Here's how the part is built. I have some questions about the finished solid (model axes, mm). A direction names the side the tool comes from. Coordinates: 2 decimals unless noted, no trailing zeros. Write each loop counter-clockwise with the first axis right and the second up, starting at its lowest first coordinate (ties: lowest second). Pieces come first, ordered by that corner, then holes. Notation, with made-up numbers: M 39.5,-23 L 57.5,-23 A18 cw 57.5,5 Z; hole C -17,88 d10. An arc over 180 degrees is marked long. Use a Markdown table: item, result.
```python
from build123d import *

# Parameters (mm, degrees)
F0_R     = 25
F0_R_2   = 5
F0_R_3   = 2.5
F0_R_4   = 3.5
F1_DEPTH = 19
F2_T     = -4
F3_DEPTH = 25
F4_R     = 25
F5_DEPTH = 2


# Not quite as in the source:
# - a feature names something its author has since deleted; it is built from what else it names


with BuildPart() as f1:
    # F0 (on Top) → F1 (new body)
    with BuildSketch(Plane.XY):
        Circle(F0_R)
        with Locations((-12.990381, -7.5)):
            Circle(F0_R_2, mode=Mode.SUBTRACT)
        with Locations((0, -15)):
            Circle(F0_R_3, mode=Mode.SUBTRACT)
        with Locations((12.990381, -7.5)):
            Circle(F0_R_2, mode=Mode.SUBTRACT)
        with Locations((-12.990381, 7.5)):
            Circle(F0_R_3, mode=Mode.SUBTRACT)
        Circle(F0_R_4, mode=Mode.SUBTRACT)
        with Locations((12.990381, 7.5)):
            Circle(F0_R_3, mode=Mode.SUBTRACT)
        with Locations((0, 15)):
            Circle(F0_R_2, mode=Mode.SUBTRACT)
        Circle(F0_R_4)
        with Locations((-12.990381, 7.5)):
            Circle(F0_R_3)
        with Locations((12.990381, 7.5)):
            Circle(F0_R_3)
        with Locations((0, -15)):
            Circle(F0_R_3)
    extrude(amount=F1_DEPTH)

    # F2
    f2_openings = [f1.faces().sort_by_distance(p)[0] for p in [
        (0, 0, 19),
    ]]
    offset(amount=F2_T, openings=f2_openings)

    # F0 (on Top) → F3 (cut)
    with BuildSketch(Plane.XY):
        with Locations((-12.990381, 7.5)):
            Circle(F0_R_3)
        Circle(F0_R_4)
        with Locations((12.990381, 7.5)):
            Circle(F0_R_3)
        with Locations((0, -15)):
            Circle(F0_R_3)
    extrude(amount=F3_DEPTH, mode=Mode.SUBTRACT)

    # F4 (on face) → F5 (join)
    with BuildSketch(Plane.XY.offset(19)):
        Circle(F4_R)
        with BuildLine():
            ThreePointArc((-20.78461, -3), (-18.186533, 10.5), (-7.794229, 19.5))
            ThreePointArc((-7.794229, 19.5), (0, 6), (7.794229, 19.5))
            ThreePointArc((7.794229, 19.5), (18.186533, 10.5), (20.78461, -3))
            ThreePointArc((20.78461, -3), (5.196152, -3), (12.990381, -16.5))
            ThreePointArc((12.990381, -16.5), (0, -21), (-12.990381, -16.5))
            ThreePointArc((-12.990381, -16.5), (-5.196152, -3), (-20.78461, -3))
        make_face(mode=Mode.SUBTRACT)
    extrude(amount=F5_DEPTH)


solid = f1.part
```
1. I need wall thicknesses on probe 1 along Y at (x, z) = (0, 1); probe 2 along Y at (x, z) = (14.5, 12.5); probe 3 along Y at (x, z) = (14, 1.5). Which ranges of each line are inside material? Lowest first, please.
Answers follow:
| item | result |
|---|---|
| probe 1 | y = -25 to -17.5, -12.5 to -3.5, 3.5 to 10, 20 to 25 |
| probe 2 | y = -20.37 to -12.27, -2.73 to 1.37, 15.19 to 20.37 |
| probe 3 | y = -20.71 to -12.4, -2.6 to 5.21, 9.79 to 20.71 |
2. Suppose I cut it at D-D on y = 7.5. Write out the boundary of the cut face in (x, z), and give its area (3 significant figures).
Answers follow:
| item | result |
|---|---|
| outline | M -23.85,0 L -15.49,0 L -15.49,4 L -19.62,4 L -19.62,21 L -23.85,21 Z; M -10.49,0 L 10.49,0 L 10.49,4 L 4.97,4 L 4.97,21 L -4.97,21 L -4.97,4 L -10.49,4 Z; M 15.49,0 L 23.85,0 L 23.85,21 L 19.62,21 L 19.62,4 L 15.49,4 Z |
| area | 464 mm2 |
3. We'd pull the mould along X, two halves only. Please class faces 1 (the face through (12.45, 5.06, 1.97)), 2 (the face through (12.339, -2.543, 9.367)), 3 (the face through (5, 0, 0)), 4 (the face through (23.846, 7.509, 10.353)): +X half, -X half, draft (parallel to the pull), parting line (faces both ways), or undercut.
Answers follow:
| item | result |
|---|---|
| face 1 | undercut |
| face 2 | undercut |
| face 3 | draft |
| face 4 | parting line |
4. Suppose I cut it at C-C on y = -15. Write out the boundary of the cut face in (x, z), and give its area (3 significant figures).
Answers follow:
| item | result |
|---|---|
| outline | M -20,0 L -2.5,0 L -2.5,4 L -8.02,4 L -8.02,21 L -20,21 Z; M 2.5,0 L 20,0 L 20,21 L 8.02,21 L 8.02,4 L 2.5,4 Z |
| area | 547 mm2 |
5. Suppose I cut it at A-A on z = 8.5. Write out the boundary of the cut face in (x, y), and give its area (3 significant figures).
Answers follow:
| item | result |
|---|---|
| outline | C 0,0 d50; hole M -20.78,-3 A9 cw long -12.99,-16.5 A21 ccw 12.99,-16.5 A9 cw long 20.78,-3 A21 ccw 7.79,19.5 A9 cw long -7.79,19.5 A21 ccw Z; hole C -12.99,-7.5 d10; hole C 0,15 d10; hole C 12.99,-7.5 d10 |
| area | 1,000 mm2 |
6. Which directions (+Z, -Z, +X, -X, +Y, -Y) give clear straight access to the entire face, cutting with the end or side of a thin tool? Please do faces 5 (the face through (3.233, -1.341, 1.972)), 6 (the face through (0, 4, 4)), 7 (the face through (-13, -7, 19)).
Answers follow:
| item | result |
|---|---|
| face 5 | +Z, -Z |
| face 6 | +Z |
| face 7 | -Z |
7. Suppose I cut it at B-B on x = -0.5. Write out the boundary of the cut face in (y, z) (3 decimals).
Answers follow:
| item | result |
|---|---|
| outline | M -24.995,0 L -17.449,0 L -17.449,4 L -20.994,4 L -20.994,21 L -24.995,21 Z; M -12.551,0 L -3.464,0 L -3.464,4 L -12.551,4 Z; M 3.464,0 L 10.025,0 L 10.025,19 L 19.975,19 L 19.975,0 L 24.995,0 L 24.995,21 L 6.014,21 L 6.014,4 L 3.464,4 Z |
8. Will these pins go through, and if not, where does the flat tip stop? pin 1 Ø5 at (x, z) = (-16.5, 13.5) entering from +Y; pin 2 Ø5 at (y, z) = (-5, 10) entering from +X; pin 3 Ø1.5 at (x, z) = (19, 13) entering from -Y; pin 4 Ø20 at (x, y) = (3, -4.5) entering from +Z.
Answers follow:
| item | result |
|---|---|
| pin 1 | stops at y = 20.71 |
| pin 2 | stops at x = 24.87 |
| pin 3 | stops at y = -17.09 |
| pin 4 | stops at z = 21 |
